```python
from build123d import *

# Parameters (mm, degrees)
F0_W     = 16.1397904158
F0_H     = 70.5894511193
F1_DEPTH = 7.62
F2_R     = 5.08
F3_R     = 5.08
F4_R     = 5.08
F5_R     = 5.08
F6_T     = 2.54


with BuildPart() as f1:
    # F0 (on Top) → F1 (new body)
    with BuildSketch(Plane.XY):
        with Locations((-135.1853534579, 5.979702808)):
            Rectangle(F0_W, F0_H)
    extrude(amount=F1_DEPTH)

    # F2
    f2_edges = [f1.edges().sort_by_distance(p)[0] for p in [
        (-143.255249, -29.315023, 3.81),
    ]]
    fillet(f2_edges, radius=F2_R)

    # F3
    f3_edges = [f1.edges().sort_by_distance(p)[0] for p in [
        (-127.115458, -29.315023, 3.81),
    ]]
    fillet(f3_edges, radius=F3_R)

    # F4
    f4_edges = [f1.edges().sort_by_distance(p)[0] for p in [
        (-143.255249, 41.274428, 3.81),
    ]]
    fillet(f4_edges, radius=F4_R)

    # F5
    f5_edges = [f1.edges().sort_by_distance(p)[0] for p in [
        (-127.115458, 41.274428, 3.81),
    ]]
    fillet(f5_edges, radius=F5_R)

    # F6
    f6_openings = [f1.faces().sort_by_distance(p)[0] for p in [
        (-135.185353, 5.979703, 7.62),
    ]]
    offset(amount=F6_T, openings=f6_openings, kind=Kind.INTERSECTION)


solid = f1.part
```
For this review, take the finished solid that the model builds, in its own axes (mm). A direction names the side the tool comes from. Give positions to 0.01 mm unless a question says otherwise; leave off trailing zeros. Write each loop counter-clockwise with the first axis right and the second up, starting at its lowest first coordinate (ties: lowest second). Pieces come first, ordered by that corner, then holes. Notation, with made-up numbers: M -16,23.25 L 10,23.25 A6 cw 10,33.25 Z; hole C 12.25,72.25 d8. An arc over 180 degrees is marked long. Answer as a JSON object with one key per item and string values. Group by question number.
Item 1: Draft analysis for pull direction Y (two halves, no side actions). For faces 1 (the flat face through (-135, 6, 0)), 2 (the cylindrical face through (-126.867, -29.682, 2.611)), 3 (the flat face through (-124.575, 6, 2)), state which applies: +Y half, -Y half, draft (parallel to the pull), parting line (faces both ways), or undercut.
Item 2: Consider section B-B on x = -137. Write out the cut boundary in (y, z), plus the area to 3 significant figures.
Item 3: For probe 1 along X at (y, z) = (2, 7.25); probe 2 along Y at (x, z) = (-132.75, 5.25); probe 3 along Y at (x, z) = (-141.75, 1), list the stretches that pass through material, from the lowest coordinate up. Write a range as [from, to].
Item 4: For pin 1 Ø1.5 at (x, y) = (-142, 11) entering from +Z; pin 2 Ø4 at (x, z) = (-130.5, 4.5) entering from -Y (3 decimals), all flat-tipped, find the tip position at first contact; note any pin that passes through.
Item 5: Consider section D-D on x = -144. Write out the cut boundary in (y, z).
Item 6: Consider section C-C on z = -1. Write out the cut boundary in (x, y), plus the area to 3 significant figures.
Item 7: Tool access review of faces 4 (the cylindrical face through (-128.643, 39.826, 3.863)), 5 (the cylindrical face through (-143.622, 41.523, 2.611)): name each direction out of +Z, -Z, +X, -X, +Y, -Y from which nothing blocks a thin tool from reaching the whole face with its end or side.
Item 8: Consider section A-A on z = 6.5. Write out the cut boundary in (x, y), plus the area to 3 significant figures.
Check result:
{
 "1": {"face 1": "undercut", "face 2": "-Y half", "face 3": "draft"},
 "2": {"outline": "M -31.86,-2.54 L 43.81,-2.54 L 43.81,7.62 L 41.27,7.62 L 41.27,0 L -29.32,0 L -29.32,7.62 L -31.86,7.62 Z", "area": "231 mm^2"},
 "3": {"probe 1": "x = [-145.8, -143.26], [-127.12, -124.58]", "probe 2": "y = [-31.86, -29.32], [41.27, 43.81]", "probe 3": "y = [-30.96, -27.84], [39.8, 42.92]"},
 "4": {"pin 1": "stops at z = 0", "pin 2": "stops at y = -31.855"},
 "5": {"outline": "M -29.15,-2.54 L 41.11,-2.54 L 41.11,7.62 L -29.15,7.62 Z"},
 "6": {"outline": "M -145.8,-24.24 A7.62 ccw -138.18,-31.86 L -132.2,-31.86 A7.62 ccw -124.58,-24.24 L -124.58,36.19 A7.62 ccw -132.2,43.81 L -138.18,43.81 A7.62 ccw -145.8,36.19 Z", "area": "1,560 mm^2"},
 "7": {"face 4": "+Z", "face 5": "+Z, -Z, -X, +Y"},
 "8": {"outline": "M -145.8,-24.24 A7.62 ccw -138.18,-31.86 L -132.2,-31.86 A7.62 ccw -124.58,-24.24 L -124.58,36.19 A7.62 ccw -132.2,43.81 L -138.18,43.81 A7.62 ccw -145.8,36.19 Z; hole M -143.26,-24.24 A5.08 ccw -138.18,-29.32 L -132.2,-29.32 A5.08 ccw -127.12,-24.24 L -127.12,36.19 A5.08 ccw -132.2,41.27 L -138.18,41.27 A5.08 ccw -143.26,36.19 Z", "area": "439 mm^2"}
}
